from build123d import *

# Parameters (mm, degrees)
F2_W     = 100
F2_H     = 100
F2_R     = 40
F3_DEPTH = 12


with BuildPart() as f1:
    # F0 (on Front) → F1 (revolve)
    with BuildSketch(Plane.XZ):
        Polygon((-40, 0), (-17.5, 0), (-17.5, 5), (-20, 11), (-20.5, 11), (-20.5, 12), (-40, 12), align=None)
    revolve(axis=Axis((0, 0, 25.371263), (0, 0, 1)))

    # F2 (on face) → F3 (join)
    with BuildSketch(Plane.XY.offset(12)):
        Rectangle(F2_W, F2_H)
        Circle(F2_R, mode=Mode.SUBTRACT)
    extrude(amount=-F3_DEPTH)


solid = f1.part
For this review, take the finished solid that the model builds, in its own axes (mm). A direction names the side the tool comes from. Round coordinates to 2 decimals unless told otherwise and drop trailing zeros. Loops run counter-clockwise (first coordinate to the right, second up) from the corner with the lowest first, then second, coordinate; pieces in that order, holes last. Notation, with made-up numbers: (21, 39.5) - (39, 39.5) arc R12 ccw to (39, 44.5) - close; hole circle Ø8 at (77.5, -22). An arc over 180 degrees is marked (long way). One line per item, written item: value. Start each with the question number.
Item 1: For faces 1 (the flat face through (18.1, 9, 11)), 2 (the flat face through (-1, 23, 12)), list the 3-axis set-ups (+Z, -Z, +X, -X, +Y, -Y) from which the entire face can be reached by the end or side of a thin tool; tool diameter is ignored.
Item 2: Take a section at C-C (z = 8). Give the boundary of the cut face in (x, y), plus the area to 3 significant figures.
Item 3: Take a section at A-A (y = 0). Give the boundary of the cut face in (x, z), plus the area to 3 significant figures.
Item 4: The part is to be moulded in two halves that separate along Y. For faces 3 (the flat face through (-1, 23, 0)), 4 (the cylindrical face through (13.887, 10.648, 2.535)), 5 (the flat face through (-1, -50, 6)), say which applies: +Y half, -Y half, draft (parallel to the pull), parting line (faces both ways), or undercut.
Item 5: For L1, parallel to Y at x = 0, z = 2.9; L2, parallel to X at y = 0, z = 11.8, list the stretches that pass through material, from the lowest coordinate up.
Answer below:
1. face 1: +Z
1. face 2: +Z, +X, -X, +Y, -Y
2. outline: (-50, -50) - (50, -50) - (50, 50) - (-50, 50) - close; hole circle Ø37.5 at (0, 0)
2. area: 8,900 mm2
3. outline: (-50, 0) - (-17.5, 0) - (-17.5, 5) - (-20, 11) - (-20.5, 11) - (-20.5, 12) - (-50, 12) - close; (17.5, 0) - (50, 0) - (50, 12) - (20.5, 12) - (20.5, 11) - (20, 11) - (17.5, 5) - close
3. area: 759 mm2
4. face 3: draft
4. face 4: undercut
4. face 5: -Y half
5. L1: y = -50 to -17.5, 17.5 to 50
5. L2: x = -50 to -20.5, 20.5 to 50
